Geometry check sheet. Reference: the model listing, model coordinates, mm. Face numbers are marked on the shaded views. A direction names the side the tool comes from. Give positions to 0.01 mm unless a question says otherwise; leave off trailing zeros. Order: outer loops, then holes, each group sorted by start corner. A loop starts at its lowest first (then second) coordinate and runs counter-clockwise, first axis right, second up.
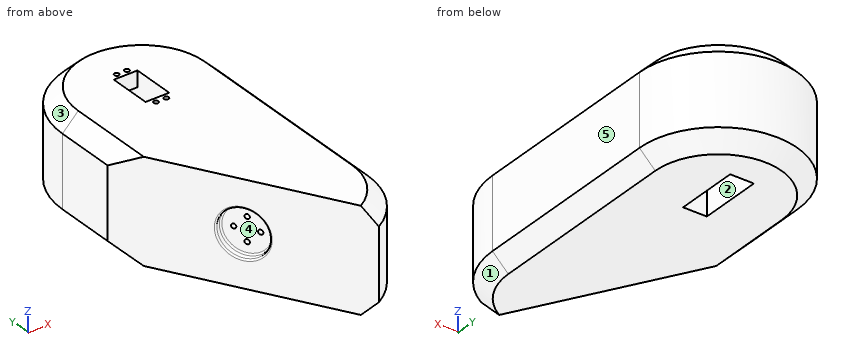
from build123d import *

# Parameters (mm, degrees)
BOSS_EXTRUDE1_DEPTH = 65
CUT_EXTRUDE1_DEPTH  = 194.261480901
SKETCH5_R           = 15
CUT_EXTRUDE4_DEPTH  = 5
SKETCH6_R           = 1.5
CUT_EXTRUDE5_DEPTH  = 7.5
CHAMFER1_SIZE       = 10
SKETCH8_W           = 15
SKETCH8_H           = 40
CUT_EXTRUDE6_DEPTH  = 55
SKETCH9_W           = 15
SKETCH9_H           = 27
SKETCH9_R           = 1.5
CUT_EXTRUDE7_DEPTH  = 191.131533418
FILLET1_R           = 1


with BuildPart() as part:
    # Sketch1 → Boss-Extrude1 (new body)
    with BuildSketch(Plane.XY):
        with BuildLine():
            Line((-50, 125), (-50, 0))
            ThreePointArc((-50, 0), (0, -50), (50, 0))
            Line((50, 0), (50, 125))
            ThreePointArc((50, 125), (0, 175), (-50, 125))
        make_face()
    extrude(amount=BOSS_EXTRUDE1_DEPTH)

    # Sketch2 → Cut-Extrude1 (cut, through all)
    with BuildSketch(Plane.XY.offset(65)):
        Polygon((260.825571734, -451.763142156), (25, -43.301270189), (-50, 86.602540378), (-50, 0), (-50, -471.651143468), (10.233499812, -1413.028395178), (321.059071546, -1393.140393866), align=None)
    extrude(amount=-CUT_EXTRUDE1_DEPTH, mode=Mode.SUBTRACT)

    # Sketch5 → Cut-Extrude4 (cut)
    with BuildSketch(Plane(origin=(0, 0, 0), x_dir=(0, 0, 1), z_dir=(-0.866025403784438, -0.5000000000000012, 0))):
        with Locations(Location((32.5, 25, 0), (0, 0, 270))):
            Circle(SKETCH5_R)
    extrude(amount=-CUT_EXTRUDE4_DEPTH, mode=Mode.SUBTRACT)

    # Sketch6 → Cut-Extrude5 (cut)
    with BuildSketch(Plane(origin=(4.330127019, 2.5, 0), x_dir=(0, 0, 1), z_dir=(-0.8660254037844378, -0.5000000000000012, 0))):
        with Locations(Location((40, 25, 0), (0, 0, 270))):
            Circle(SKETCH6_R)
        with Locations(Location((32.5, 32.5, 0), (0, 0, 270))):
            Circle(SKETCH6_R)
        with Locations(Location((32.5, 17.5, 0), (0, 0, 270))):
            Circle(SKETCH6_R)
        with Locations(Location((25, 25, 0), (0, 0, 270))):
            Circle(SKETCH6_R)
    extrude(amount=-CUT_EXTRUDE5_DEPTH, mode=Mode.SUBTRACT)

    # Chamfer1
    chamfer1_edges = [part.edges().sort_by_distance(p)[0] for p in [
        (43.301270189, -25, 0),
        (43.301270189, -25, 65),
        (50, 62.5, 65),
        (0, 175, 65),
        (50, 62.5, 0),
        (-50, 105.801270189, 0),
        (0, 175, 0),
        (-50, 105.801270189, 65),
    ]]
    chamfer(chamfer1_edges, length=CHAMFER1_SIZE)

    # Sketch8 → Cut-Extrude6 (cut)
    with BuildSketch(Plane(origin=(0, 0, 0), x_dir=(-1, 0, 0), z_dir=(0, 0, -1))):
        with Locations((0, 125)):
            Rectangle(SKETCH8_W, SKETCH8_H)
    extrude(amount=-CUT_EXTRUDE6_DEPTH, mode=Mode.SUBTRACT)

    # Sketch9 → Cut-Extrude7 (cut, through all)
    with BuildSketch(Plane(origin=(0, 0, 55), x_dir=(-1, 0, 0), z_dir=(0, 0, -1))):
        with Locations((0, 125)):
            Rectangle(SKETCH9_W, SKETCH9_H)
        with Locations((-3.25, 108.25)):
            Circle(SKETCH9_R)
        with Locations((3.25, 108.25)):
            Circle(SKETCH9_R)
        with Locations((-3.25, 141.75)):
            Circle(SKETCH9_R)
        with Locations((3.25, 141.75)):
            Circle(SKETCH9_R)
    extrude(amount=-CUT_EXTRUDE7_DEPTH, mode=Mode.SUBTRACT)

    # Fillet1
    fillet1_edges = [part.edges().sort_by_distance(p)[0] for p in [
        (-15.669872981, 37.141016151, 32.5),
        (-20, 34.641016151, 32.5),
    ]]
    fillet(fillet1_edges, radius=FILLET1_R)


solid = part.part
Item 1: Sectioned sample at C-C (z = 8). Enter the section's corners in (x, y).
Reported:
outline: (-48, 83.14) - (24, -41.57) arc R48 ccw to (48, 0) - (48, 125) arc R48 ccw to (-48, 125) - close; hole (-7.5, 105) - (7.5, 105) - (7.5, 145) - (-7.5, 145) - close
Item 2: Sectioned sample at A-A (z = 52.5). Enter the section's corners in (x, y).
Reported:
outline: (-50, 86.6) - (25, -43.3) arc R50 ccw to (50, 0) - (50, 125) arc R50 ccw to (-50, 125) - close; hole (-7.5, 105) - (7.5, 105) - (7.5, 145) - (-7.5, 145) - close
Item 3: Draft check along Z on the marked faces 3, 4 and 5. Enter one of: released by +Z, released by -Z, zero draft, split by the parting line, or undercut.
Reported:
face 3: released by +Z
face 4: undercut
face 5: zero draft
Item 4: Scan lines: L1, parallel to X at y = 141.75, z = 60; L2, parallel to Y at x = -3.25, z = 59.25; L3, parallel to Y at x = -3, z = 59. Record each from-to range of solid material in increasing order.
Reported:
L1: x = -41.77 to -4.75, -1.75 to 1.75, 4.75 to 41.77
L2: y = 5.63 to 106.75, 109.75 to 111.5, 138.5 to 140.25, 143.25 to 170.63
L3: y = 5.2 to 106.77, 109.73 to 111.5, 138.5 to 140.27, 143.23 to 170.9
Item 5: Set-up check for the marked faces 1 and 2: record each of +Z, -Z, +X, -X, +Y, -Y from which the full face is reachable in a straight line by a thin tool's end or side.
Reported:
face 1: -Z, +X, -Y
face 2: -Z
Item 6: Gauge pin test, flat ends, axial feed: pin 1 (5 mm diameter, centred on x = 39.5, z = 13, fed in from -Y); pin 2 (3 mm diameter, centred on x = -0.5, y = 108.5, fed in from -Z); pin 3 (3 mm diameter, centred on y = -7.5, z = 57.5, fed in from +X). Record the tip position at first contact, or that the pin passes through.
Reported:
pin 1: stops at y = -33.63
pin 2: stops at z = 55
pin 3: stops at x = 48.44
Item 7: Sectioned sample at B-B (y = 3.5). Enter the section's corners in (x, z), and give its area (3 significant figures).
Reported:
outline: (-2.02, 0) - (40, 0) - (50, 10) - (50, 55) - (40, 65) - (-2.02, 65) - close
area: 3,280 mm2
